```python
from build123d import *

# Parameters (mm, degrees)
SKETCH1_R           = 2.5
BOSS_EXTRUDE1_DEPTH = 3.5
SKETCH2_R           = 1.5
CUT_EXTRUDE1_DEPTH  = 77.148499601
FILLET1_R           = 10
SKETCH3_R           = 15.25
SKETCH3_R_2         = 3
CUT_EXTRUDE2_DEPTH  = 77.148499601


with BuildPart() as part:
    # Sketch1 → Boss-Extrude1 (new body)
    with BuildSketch(Plane.XY):
        with BuildLine():
            Line((0, -19), (30, -19))
            Line((30, -19), (64.201367261, 15.201367261))
            Line((64.201367261, 15.201367261), (58.615223689, 20.787510832))
            Line((58.615223689, 20.787510832), (44.190245353, 35.212489168))
            Line((44.190245353, 35.212489168), (38.604101782, 40.798632739))
            Line((38.604101782, 40.798632739), (16.805469042, 19))
            Line((16.805469042, 19), (0, 19))
            ThreePointArc((0, 19), (-19, 0), (0, -19))
        make_face()
        Circle(SKETCH1_R, mode=Mode.SUBTRACT)
    extrude(amount=BOSS_EXTRUDE1_DEPTH)

    # Sketch2 → Cut-Extrude1 (cut, through all)
    with BuildSketch(Plane.XY.offset(3.5)):
        with Locations((38.878105659, 35.574881393)):
            Circle(SKETCH2_R)
        with Locations((58.977615915, 15.475371138)):
            Circle(SKETCH2_R)
    extrude(amount=-CUT_EXTRUDE1_DEPTH, mode=Mode.SUBTRACT)

    # Fillet1
    fillet1_edges = [part.edges().sort_by_distance(p)[0] for p in [
        (16.805469042, 19, 1.75),
        (30, -19, 1.75),
    ]]
    fillet(fillet1_edges, radius=FILLET1_R)

    # Sketch3 → Cut-Extrude2 (cut, through all)
    with BuildSketch(Plane.XY.offset(3.5)):
        Circle(SKETCH3_R)
        with Locations((38.878105659, 35.574881393)):
            Circle(SKETCH3_R_2)
        with Locations((58.977615915, 15.475371138)):
            Circle(SKETCH3_R_2)
    extrude(amount=-CUT_EXTRUDE2_DEPTH, mode=Mode.SUBTRACT)


solid = part.part
```
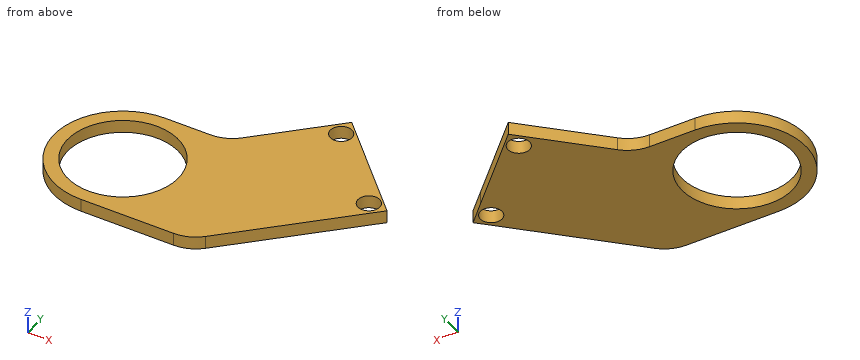
Check sheet for the modelled part. Datum: model origin and axes. Units: mm. Give positions to 0.01 mm unless a question says otherwise; leave off trailing zeros. Order: outer loops, then holes, each group sorted by start corner. A loop starts at its lowest first (then second) coordinate and runs counter-clockwise, first axis right, second up. Notation, with made-up numbers: M -40,72 L -23,72 A11 ccw -23,92 Z; hole C -3.5,39 d10. An arc over 180 degrees is marked long. Answer in a Markdown table with one row per item. Add a question column.
Q1. Sectioned sample at D-D, the plane x = 24.5. Record the boundary of the cut face in (y, z), and give its area (3 significant figures).
Q2. Sectioned sample at C-C, the plane z = 1.2. Record the boundary of the cut face in (x, y), and give its area (3 significant figures).
Q3. Sectioned sample at B-B, the plane x = 37. Record the boundary of the cut face in (y, z).
Q4. Sectioned sample at A-A, the plane y = 0. Record the boundary of the cut face in (x, z), and give its area (3 significant figures).
Q5. Thickness scan on L1, parallel to Y at x = 0, z = 2.65; L2, parallel to X at y = -8, z = 2.1; L3, parallel to Y at x = -8, z = 1.35. Record the ranges inside material, lowest first.
Q6. Gauge pin test, flat end, axial feed: pin 1 Ø2 at (x, z) = (53, 1) entering from -Y. Record the tip position at first contact, or that the pin passes through.
Verdict:
| question | item | result |
|---|---|---|
| 1 | outline | M -19,0 L 26.69,0 L 26.69,3.5 L -19,3.5 Z |
| 1 | area | 160 mm² |
| 2 | outline | M 0,-19 L 25.86,-19 A10 ccw 32.93,-16.07 L 64.2,15.2 L 38.6,40.8 L 19.73,21.93 A10 cw 12.66,19 L 0,19 A19 ccw Z; hole C 0,0 d30.5; hole C 38.88,35.57 d6; hole C 58.98,15.48 d6 |
| 2 | area | 2,100 mm² |
| 3 | outline | M -12,0 L 33.24,0 L 33.24,3.5 L -12,3.5 Z; M 37.91,0 L 39.19,0 L 39.19,3.5 L 37.91,3.5 Z |
| 4 | outline | M -19,0 L -15.25,0 L -15.25,3.5 L -19,3.5 Z; M 15.25,0 L 49,0 L 49,3.5 L 15.25,3.5 Z |
| 4 | area | 131 mm² |
| 5 | L1 | -19 to -15.25, 15.25 to 19 |
| 5 | L2 | -17.23 to -12.98, 12.98 to 41 |
| 5 | L3 | -17.23 to -12.98, 12.98 to 17.23 |
| 6 | pin 1 | y = 3 |
